Here's how the part is built. I have some questions about the finished solid (model axes, mm). A direction names the side the tool comes from. Coordinates: 2 decimals unless noted, no trailing zeros. Write each loop counter-clockwise with the first axis right and the second up, starting at its lowest first coordinate (ties: lowest second). Pieces come first, ordered by that corner, then holes. Notation, with made-up numbers: M 67,-0.5 L 75,-0.5 A4 cw 75,4.5 Z; hole C 25.25,29.25 d7. An arc over 180 degrees is marked long. Use a Markdown table: item, result.
```python
from build123d import *

# Parameters (mm, degrees)
CYLINDER178_R          = 3
CYLINDER178_DEPTH      = 60
CYLINDER178_ROLL_ANGLE = 90
BOX109_W               = 38
BOX109_H               = 16
BOX109_DEPTH           = 16
BOX107_W               = 40
BOX107_H               = 40
BOX107_DEPTH           = 200
CYLINDER180_R          = 3
CYLINDER180_DEPTH      = 60
CYLINDER180_ROLL_ANGLE = 90
BOX110_W               = 8
BOX110_H               = 18
BOX110_DEPTH           = 60
CYLINDER179_R          = 3
CYLINDER179_DEPTH      = 60
CYLINDER179_ROLL_ANGLE = 90
BOX105_W               = 8
BOX105_H               = 18
BOX105_DEPTH           = 60
BOX106_W               = 470
BOX106_H               = 40
BOX106_DEPTH           = 40
FILLET_R               = 19
FILLET001_R            = 5
FILLET002_R            = 8


with BuildPart() as cilindro102:
    # Cylinder178 → Cylinder178 (new body)
    with BuildSketch(Plane.XY):
        Circle(CYLINDER178_R)
    extrude(amount=CYLINDER178_DEPTH)


with BuildPart() as cilindro102_1:
    # Cylinder178 roll: moved
    add(cilindro102.part.rotate(Axis((0, 0, 0), (1, 0, 0)), CYLINDER178_ROLL_ANGLE))


with BuildPart() as cilindro102_2:
    # Cylinder178 placement: moved
    add(cilindro102_1.part.moved(Location((5, 37, 765))))


with BuildPart() as cubo075:
    # Box109 → Box109 (new body)
    with BuildSketch(Plane(origin=(-10, -8, 756), x_dir=(1, 0, 0), z_dir=(0, 0, 1))):
        with Locations((19, 8)):
            Rectangle(BOX109_W, BOX109_H)
    extrude(amount=BOX109_DEPTH)


with BuildPart() as cut001:
    # Box107 → Box107 (new body)
    with BuildSketch(Plane(origin=(-50, -20, 585), x_dir=(1, 0, 0), z_dir=(0, 0, 1))):
        with Locations((20, 20)):
            Rectangle(BOX107_W, BOX107_H)
    extrude(amount=BOX107_DEPTH)

    # Fusion054: union Cubo075
    add(cubo075.part)

    # Cut220: cut Cilindro102
    add(cilindro102_2.part, mode=Mode.SUBTRACT)


with BuildPart() as cilindro104:
    # Cylinder180 → Cylinder180 (new body)
    with BuildSketch(Plane.XY):
        Circle(CYLINDER180_R)
    extrude(amount=CYLINDER180_DEPTH)


with BuildPart() as cilindro104_1:
    # Cylinder180 roll: moved
    add(cilindro104.part.rotate(Axis((0, 0, 0), (1, 0, 0)), CYLINDER180_ROLL_ANGLE))


with BuildPart() as cilindro104_2:
    # Cylinder180 placement: moved
    add(cilindro104_1.part.moved(Location((-18, 30, 532))))


with BuildPart() as obj1:
    # Box110 → Box110 (new body)
    with BuildSketch(Plane(origin=(-22, -9, 525), x_dir=(1, 0, 0), z_dir=(0, 0, 1))):
        with Locations((4, 9)):
            Rectangle(BOX110_W, BOX110_H)
    extrude(amount=BOX110_DEPTH)

    # Cut222: cut Cilindro104
    add(cilindro104_2.part, mode=Mode.SUBTRACT)


with BuildPart() as obj1_1:
    # Cut222 placement: moved
    add(obj1.part.moved(Location((-454, 0, 0))))


with BuildPart() as cilindro103:
    # Cylinder179 → Cylinder179 (new body)
    with BuildSketch(Plane.XY):
        Circle(CYLINDER179_R)
    extrude(amount=CYLINDER179_DEPTH)


with BuildPart() as cilindro103_1:
    # Cylinder179 roll: moved
    add(cilindro103.part.rotate(Axis((0, 0, 0), (1, 0, 0)), CYLINDER179_ROLL_ANGLE))


with BuildPart() as cilindro103_2:
    # Cylinder179 placement: moved
    add(cilindro103_1.part.moved(Location((-18, 30, 532))))


with BuildPart() as cut221:
    # Box105 → Box105 (new body)
    with BuildSketch(Plane(origin=(-22, -9, 525), x_dir=(1, 0, 0), z_dir=(0, 0, 1))):
        with Locations((4, 9)):
            Rectangle(BOX105_W, BOX105_H)
    extrude(amount=BOX105_DEPTH)

    # Cut221: cut Cilindro103
    add(cilindro103_2.part, mode=Mode.SUBTRACT)


with BuildPart() as cut221_1:
    # Cut221 placement: moved
    add(cut221.part.moved(Location((0, 0, 5))))


with BuildPart() as fillet002:
    # Box106 → Box106 (new body)
    with BuildSketch(Plane(origin=(-480, -20, 585), x_dir=(1, 0, 0), z_dir=(0, 0, 1))):
        with Locations((235, 20)):
            Rectangle(BOX106_W, BOX106_H)
    extrude(amount=BOX106_DEPTH)

    # Fusion055: union obj1, Cut221
    add(obj1_1.part)
    add(cut221_1.part)

    # Fusion059: union cut001
    add(cut001.part)


with BuildPart() as fillet002_1:
    # Fusion059 placement: moved
    add(fillet002.part.moved(Location((0, 460, 0))))

    # Fillet
    fillet_edges = [fillet002_1.edges().sort_by_distance(p)[0] for p in [
        (-30, 480, 785),
        (-30, 440, 785),
    ]]
    fillet(fillet_edges, radius=FILLET_R)

    # Fillet001
    fillet001_edges = [fillet002_1.edges().sort_by_distance(p)[0] for p in [
        (-50, 460, 625),
    ]]
    fillet(fillet001_edges, radius=FILLET001_R)

    # Fillet002
    fillet002_edges = [fillet002_1.edges().sort_by_distance(p)[0] for p in [
        (-480, 460, 625),
    ]]
    fillet(fillet002_edges, radius=FILLET002_R)


solid = fillet002_1.part
```
1. I need wall thicknesses on probe 1 along X at (y, z) = (457, 532); probe 2 along X at (y, z) = (461, 537); probe 3 along Z at (x, y) = (5, 456). Which ranges of each line are inside material? Lowest first, please.
Answers follow:
| item | result |
|---|---|
| probe 1 | x = -476 to -475, -469 to -468, -22 to -14 |
| probe 2 | x = -476 to -468, -22 to -21, -15 to -14 |
| probe 3 | z = 756 to 762, 768 to 772 |
2. Which directions (+Z, -Z, +X, -X, +Y, -Y) give clear straight access to the entire face, cutting with the end or side of a thin tool? Please do faces 5 (the face through (9, 452, 764)), 6 (the face through (9, 468, 764)), 7 (the face through (-476, 460, 555)).
Answers follow:
| item | result |
|---|---|
| face 5 | +Z, -Z, +X, -Y |
| face 6 | +Z, -Z, +X, +Y |
| face 7 | -Z, -X, +Y, -Y |
3. Suppose I cut it at B-B on x = -107. Write out the boundary of the cut face in (y, z), and give its area (3 significant figures).
Answers follow:
| item | result |
|---|---|
| outline | M 440,585 L 480,585 L 480,625 L 440,625 Z |
| area | 1,600 mm2 |
4. Suppose I cut it at C-C on z = 672.5. Write out the boundary of the cut face in (x, y).
Answers follow:
| item | result |
|---|---|
| outline | M -50,440 L -10,440 L -10,480 L -50,480 Z |
5. Suppose I cut it at A-A on z = 576. Write out the boundary of the cut face in (x, y).
Answers follow:
| item | result |
|---|---|
| outline | M -476,451 L -468,451 L -468,469 L -476,469 Z; M -22,451 L -14,451 L -14,469 L -22,469 Z |
6. We'd pull the mould along X, two halves only. Please class faces 1 (the face through (28, 460, 764)), 2 (the face through (9, 460, 772)), 3 (the face through (-22, 460, 557)), 4 (the face through (-248, 460, 585)): +X half, -X half, draft (parallel to the pull), parting line (faces both ways), or undercut.
Answers follow:
| item | result |
|---|---|
| face 1 | +X half |
| face 2 | draft |
| face 3 | undercut |
| face 4 | undercut |
7. Will these pins go through, and if not, where does the flat tip stop? pin 1 Ø4 at (x, z) = (-18.5, 546.5) entering from -Y; pin 2 Ø9.5 at (x, z) = (-472, 532) entering from +Y; pin 3 Ø12 at (x, y) = (-84, 469) entering from +Z.
Answers follow:
| item | result |
|---|---|
| pin 1 | stops at y = 451 |
| pin 2 | stops at y = 469 |
| pin 3 | stops at z = 625 |
